Geometry check sheet. Reference: the model listing, model coordinates, mm. A direction names the side the tool comes from. Give positions to 0.01 mm unless a question says otherwise; leave off trailing zeros. Write each loop counter-clockwise with the first axis right and the second up, starting at its lowest first coordinate (ties: lowest second). Pieces come first, ordered by that corner, then holes. Notation, with made-up numbers: M 25,28.25 L 45,28.25 A18 cw 45,44.25 Z; hole C 20.5,-26.5 d11. An arc over 180 degrees is marked long. Write each question's results on one line, items separated by ' | '.
```python
from build123d import *

# Parameters (mm, degrees)
F0_W     = 77.7875
F0_H     = 98.425
F1_DEPTH = 28.575
F2_W     = 104.775
F2_H     = 44.45
F3_DEPTH = 3.175
F4_W     = 38.1
F4_H     = 28.575
F5_DEPTH = 60.325


with BuildPart() as f1:
    # F0 (on Top) → F1 (new body)
    with BuildSketch(Plane.XY):
        Rectangle(F0_W, F0_H)
    extrude(amount=F1_DEPTH)

    # F2 (on face) → F3 (join)
    with BuildSketch(Plane(origin=(0, 0, 0), x_dir=(1, 0, 0), z_dir=(0, 0, -1))):
        with Locations((0, 3.175)):
            Rectangle(F2_W, F2_H)
        with BuildLine():
            ThreePointArc((-47.625, 1.918831), (-48.211274, 8.876744), (-42.06875, 5.55625))
            ThreePointArc((-42.06875, 5.55625), (-42.717006, 3.382476), (-44.45, 1.918831))
            Line((-44.45, 1.918831), (-44.45, 0))
            ThreePointArc((-44.45, 0), (-46.0375, -1.5875), (-47.625, 0))
            Line((-47.625, 0), (-47.625, 1.918831))
        make_face(mode=Mode.SUBTRACT)
        with BuildLine():
            ThreePointArc((44.45, 1.918831), (43.863726, 8.876744), (50.00625, 5.55625))
            ThreePointArc((50.00625, 5.55625), (49.357994, 3.382476), (47.625, 1.918831))
            Line((47.625, 1.918831), (47.625, 0))
            ThreePointArc((47.625, 0), (46.0375, -1.5875), (44.45, 0))
            Line((44.45, 0), (44.45, 1.918831))
        make_face(mode=Mode.SUBTRACT)
    extrude(amount=-F3_DEPTH)

    # F4 (on face) → F5 (join)
    with BuildSketch(Plane.XZ.offset(49.2125)):
        with Locations((-19.84375, 14.2875)):
            Rectangle(F4_W, F4_H)
    extrude(amount=F5_DEPTH)


solid = f1.part
```
Q1. Section check A-A (z = 17.5). Enter the section's corners in (x, y), then the cut area to 3 significant figures.
Answer key:
outline: M -38.89,-109.54 L -0.79,-109.54 L -0.79,-49.21 L 38.89,-49.21 L 38.89,49.21 L -38.89,49.21 Z | area: 9,950 mm2
Q2. Access from +Z, -Z, +X, -X, +Y, -Y to the whole of each face (thin tool, end or side, straight path). Record for faces 1 (the face through (-0.794, -79, 14)), 2 (the face through (41, -3, 3.175)), 3 (the face through (-46, 19.05, 2)), 4 (the face through (-46, -25.4, 2)), 5 (the face through (46.072, 1.587, 1.565)).
Answer key:
face 1: +Z, -Z, +X, -Y | face 2: +Z, +X, +Y, -Y | face 3: +Z, -Z, -X, +Y | face 4: +Z, -Z, -X, -Y | face 5: +Z, -Z
Q3. Depth check by flat-ended pin: P1, Ø8.5, axis at y = -90, z = 18, coming from the +X side; P2, Ø1, axis at x = -42.5, z = 2, coming from the -Y side; P3, Ø2.5, axis at x = -45.5, z = 2, coming from the +Y side; P4, Ø10.5, axis at x = 46.04, y = -5.56, coming from the -Z side. Enter the tip coordinate at first touch or a pass-through.
Answer key:
P1: stops at x = -0.79 | P2: stops at y = -25.4 | P3: stops at y = 19.05 | P4: stops at z = 0
Q4. Section check B-B (y = 4.5). Enter the section's corners in (x, z) (1 decimal).
Answer key:
outline: M -52.4,0 L 52.4,0 L 52.4,3.2 L 38.9,3.2 L 38.9,28.6 L -38.9,28.6 L -38.9,3.2 L -52.4,3.2 Z
Q5. Material ranges on probe 1 along X at (y, z) = (-47, 27.25); probe 2 along X at (y, z) = (-65.5, 7.25); probe 3 along Z at (x, y) = (-39, -16.5) (3 decimals), recorded low to high. Write a range as [from, to].
Answer key:
probe 1: x = [-38.89, 38.89] | probe 2: x = [-38.89, -0.79] | probe 3: z = [0, 3.175]
Q6. Section check D-D (y = -51). Enter the section's corners in (x, z) (3 decimals), then the cut area to 3 significant figures.
Answer key:
outline: M -38.894,0 L -0.794,0 L -0.794,28.575 L -38.894,28.575 Z | area: 1,090 mm2
Q7. Section check C-C (x = 40.5). Enter the section's corners in (y, z) (3 decimals).
Answer key:
outline: M -25.4,0 L 19.05,0 L 19.05,3.175 L -25.4,3.175 Z
Q8. Release check for a two-part mould opening along Y. For faces 6 (the face through (-38.894, -29, 14)), 7 (the face through (-46.003, 1.587, 1.565)), 8 (the face through (46, -25.4, 2)) record: released by +Y, released by -Y, zero draft, split by the parting line, or undercut.
Answer key:
face 6: zero draft | face 7: undercut | face 8: released by -Y
